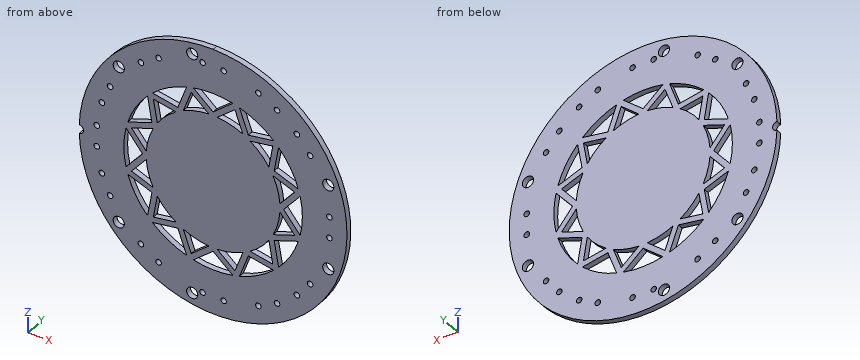
```python
from build123d import *

# Parameters (mm, degrees)
SKETCH2_R                = 88.9
BOSS_EXTRUDE1_DEPTH      = 3.175
SKETCH3_R                = 3.175
CUT_EXTRUDE1_DEPTH       = 3.175
SKETCH6_R                = 88.9
SKETCH6_R_2              = 76.2
CUT_EXTRUDE2_DEPTH       = 126.763669734
SKETCH7_R                = 1.5875
CUT_EXTRUDE3_DEPTH       = 108.809835474
SKETCH8_R                = 2.5
CUT_EXTRUDE4_DEPTH       = 108.809835474
CIRPATTERN1_COUNT        = 2
CIRPATTERN1_ANGLE        = 23
CIRPATTERN2_COUNT        = 2
CIRPATTERN2_ANGLE        = 57
CIRPATTERN3_COUNT        = 2
CIRPATTERN3_ANGLE        = 90
CIRPATTERN4_COUNT        = 2
CIRPATTERN6_COUNT        = 2
CIRPATTERN6_ANGLE        = 141
CIRPATTERN7_COUNT        = 2
CIRPATTERN7_ANGLE        = 118
MIRROR3_COPY_1_SKETCH_R  = 1.5875
MIRROR3_COPY_1_DEPTH     = 108.809835474
MIRROR3_COPY_2_SKETCH_R  = 1.5875
MIRROR3_COPY_2_DEPTH     = 108.809835474
MIRROR3_COPY_3_SKETCH_R  = 1.5875
MIRROR3_COPY_3_DEPTH     = 108.809835474
MIRROR3_COPY_4_SKETCH_R  = 1.5875
MIRROR3_COPY_4_DEPTH     = 108.809835474
MIRROR3_COPY_5_SKETCH_R  = 1.5875
MIRROR3_COPY_5_DEPTH     = 108.809835474
MIRROR3_COPY_6_SKETCH_R  = 1.5875
MIRROR3_COPY_6_DEPTH     = 108.809835474
MIRROR3_COPY_7_SKETCH_R  = 1.5875
MIRROR3_COPY_7_DEPTH     = 108.809835474
MIRROR3_COPY_8_SKETCH_R  = 1.5875
MIRROR3_COPY_8_DEPTH     = 108.809835474
MIRROR3_COPY_9_SKETCH_R  = 1.5875
MIRROR3_COPY_9_DEPTH     = 108.809835474
MIRROR3_COPY_10_SKETCH_R = 1.5875
MIRROR3_COPY_10_DEPTH    = 108.809835474
SKETCH11_R               = 50.8
SKETCH11_R_2             = 38.1
CUT_EXTRUDE6_DEPTH       = 108.809835474
EXTRUDE_THIN2_DEPTH      = 3.175


with BuildPart() as part:
    # Sketch2 → Boss-Extrude1 (new body)
    with BuildSketch(Plane(origin=(0, 0, 0), x_dir=(1, 0, 0), z_dir=(0, 1, 0))):
        with Locations(Location((0, 0, 0), (0, 0, 270))):
            Circle(SKETCH2_R)
    extrude(amount=BOSS_EXTRUDE1_DEPTH)

    # Sketch3 → Cut-Extrude1 (cut)
    with BuildSketch(Plane(origin=(0, 3.175, 0), x_dir=(1, 0, 0), z_dir=(0, 1, 0))):
        with Locations(Location((65.549718535, -24.13, 0), (0, 0, 270))):
            Circle(SKETCH3_R)
        with Locations(Location((65.549718535, 24.13, 0), (0, 0, 270))):
            Circle(SKETCH3_R)
        with Locations(Location((-53.672052261, 44.702721462, 0), (0, 0, 270))):
            Circle(SKETCH3_R)
        with Locations(Location((-11.877666274, 68.832721462, 0), (0, 0, 270))):
            Circle(SKETCH3_R)
        with Locations(Location((-11.877666274, -68.832721462, 0), (0, 0, 270))):
            Circle(SKETCH3_R)
        with Locations(Location((-53.672052261, -44.702721462, 0), (0, 0, 270))):
            Circle(SKETCH3_R)
    extrude(amount=-CUT_EXTRUDE1_DEPTH, mode=Mode.SUBTRACT)

    # Sketch6 → Cut-Extrude2 (cut, through all)
    with BuildSketch(Plane(origin=(0, 3.175, 0), x_dir=(1, 0, 0), z_dir=(0, 1, 0))):
        Circle(SKETCH6_R)
        with Locations(Location((0, 0, 0), (0, 0, 270))):
            Circle(SKETCH6_R_2, mode=Mode.SUBTRACT)
    extrude(amount=-CUT_EXTRUDE2_DEPTH, mode=Mode.SUBTRACT)

    # Sketch7 → Cut-Extrude3 (cut, symmetric)
    with BuildSketch(Plane(origin=(0, 3.175, 0), x_dir=(1, 0, 0), z_dir=(0, 1, 0))):
        with Locations(Location((-66.2, 6, 0), (0, 0, 270))):
            Circle(SKETCH7_R)
        with Locations(Location((-66.2, -6, 0), (0, 0, 270))):
            Circle(SKETCH7_R)
    cut_extrude3 = extrude(amount=CUT_EXTRUDE3_DEPTH, both=True, mode=Mode.SUBTRACT)

    # Sketch8 → Cut-Extrude4 (cut, through all)
    with BuildSketch(Plane(origin=(0, 3.175, 0), x_dir=(1, 0, 0), z_dir=(0, 1, 0))):
        with Locations((-76.2, 0)):
            Circle(SKETCH8_R)
    extrude(amount=-CUT_EXTRUDE4_DEPTH, mode=Mode.SUBTRACT)

    # CirPattern1: Cut-Extrude3 ×2 about axis
    cirpattern1_axis = Axis((0, 0, 0), (0, 1, 0))
    for i in range(1, CIRPATTERN1_COUNT):
        add(cut_extrude3.rotate(cirpattern1_axis, i * CIRPATTERN1_ANGLE / (CIRPATTERN1_COUNT - 1)), mode=Mode.SUBTRACT)

    # CirPattern2: Cut-Extrude3 ×2 about axis
    cirpattern2_axis = Axis((0, 0, 0), (0, 1, 0))
    for i in range(1, CIRPATTERN2_COUNT):
        add(cut_extrude3.rotate(cirpattern2_axis, i * CIRPATTERN2_ANGLE / (CIRPATTERN2_COUNT - 1)), mode=Mode.SUBTRACT)

    # CirPattern3: Cut-Extrude3 ×2 about axis
    cirpattern3_axis = Axis((0, 0, 0), (0, 1, 0))
    for i in range(1, CIRPATTERN3_COUNT):
        add(cut_extrude3.rotate(cirpattern3_axis, i * CIRPATTERN3_ANGLE / (CIRPATTERN3_COUNT - 1)), mode=Mode.SUBTRACT)

    # CirPattern4: Cut-Extrude3 ×2 about axis
    cirpattern4_axis = Axis((0, 0, 0), (0, 1, 0))
    for i in range(1, CIRPATTERN4_COUNT):
        add(cut_extrude3.rotate(cirpattern4_axis, i * 360 / CIRPATTERN4_COUNT), mode=Mode.SUBTRACT)

    # CirPattern6: Cut-Extrude3 ×2 about axis
    cirpattern6_axis = Axis((0, 0, 0), (0, 1, 0))
    for i in range(1, CIRPATTERN6_COUNT):
        add(cut_extrude3.rotate(cirpattern6_axis, i * CIRPATTERN6_ANGLE / (CIRPATTERN6_COUNT - 1)), mode=Mode.SUBTRACT)

    # CirPattern7: Cut-Extrude3 ×2 about axis
    cirpattern7_axis = Axis((0, 0, 0), (0, 1, 0))
    for i in range(1, CIRPATTERN7_COUNT):
        add(cut_extrude3.rotate(cirpattern7_axis, i * CIRPATTERN7_ANGLE / (CIRPATTERN7_COUNT - 1)), mode=Mode.SUBTRACT)

    # Mirror3 copy 1 sketch → Mirror3 copy 1 (cut, symmetric)
    with BuildSketch(Plane(origin=(0, 3.175, 0), x_dir=(0.9205048534524399, 0, 0.3907311284892746), z_dir=(0, 1, 0))):
        with Locations((-66.2, -6)):
            Circle(MIRROR3_COPY_1_SKETCH_R)
        with Locations((-66.2, 6)):
            Circle(MIRROR3_COPY_1_SKETCH_R)
    extrude(amount=MIRROR3_COPY_1_DEPTH, both=True, mode=Mode.SUBTRACT)

    # Mirror3 copy 2 sketch → Mirror3 copy 2 (cut, symmetric)
    with BuildSketch(Plane(origin=(0, 3.175, 0), x_dir=(1, 0, 0), z_dir=(0, 1, 0))):
        with Locations((-66.2, -6)):
            Circle(MIRROR3_COPY_2_SKETCH_R)
        with Locations((-66.2, 6)):
            Circle(MIRROR3_COPY_2_SKETCH_R)
    extrude(amount=MIRROR3_COPY_2_DEPTH, both=True, mode=Mode.SUBTRACT)

    # Mirror3 copy 3 sketch → Mirror3 copy 3 (cut, symmetric)
    with BuildSketch(Plane(origin=(0, 3.175, 0), x_dir=(0.5446390350150256, 0, 0.8386705679454249), z_dir=(0, 1, 0))):
        with Locations((-66.2, -6)):
            Circle(MIRROR3_COPY_3_SKETCH_R)
        with Locations((-66.2, 6)):
            Circle(MIRROR3_COPY_3_SKETCH_R)
    extrude(amount=MIRROR3_COPY_3_DEPTH, both=True, mode=Mode.SUBTRACT)

    # Mirror3 copy 4 sketch → Mirror3 copy 4 (cut, symmetric)
    with BuildSketch(Plane(origin=(0, 3.175, 0), x_dir=(1, 0, 0), z_dir=(0, 1, 0))):
        with Locations((-66.2, -6)):
            Circle(MIRROR3_COPY_4_SKETCH_R)
        with Locations((-66.2, 6)):
            Circle(MIRROR3_COPY_4_SKETCH_R)
    extrude(amount=MIRROR3_COPY_4_DEPTH, both=True, mode=Mode.SUBTRACT)

    # Mirror3 copy 5 sketch → Mirror3 copy 5 (cut, symmetric)
    with BuildSketch(Plane.ZX.offset(3.175)):
        with Locations((-66.2, -6)):
            Circle(MIRROR3_COPY_5_SKETCH_R)
        with Locations((-66.2, 6)):
            Circle(MIRROR3_COPY_5_SKETCH_R)
    extrude(amount=MIRROR3_COPY_5_DEPTH, both=True, mode=Mode.SUBTRACT)

    # Mirror3 copy 6 sketch → Mirror3 copy 6 (cut, symmetric)
    with BuildSketch(Plane(origin=(0, 3.175, 0), x_dir=(1, 0, 0), z_dir=(0, 1, 0))):
        with Locations((-66.2, -6)):
            Circle(MIRROR3_COPY_6_SKETCH_R)
        with Locations((-66.2, 6)):
            Circle(MIRROR3_COPY_6_SKETCH_R)
    extrude(amount=MIRROR3_COPY_6_DEPTH, both=True, mode=Mode.SUBTRACT)

    # Mirror3 copy 7 sketch → Mirror3 copy 7 (cut, symmetric)
    with BuildSketch(Plane(origin=(0, 3.175, 0), x_dir=(-0.7771459614569742, 0, 0.6293203910498333), z_dir=(0, 1, 0))):
        with Locations((-66.2, -6)):
            Circle(MIRROR3_COPY_7_SKETCH_R)
        with Locations((-66.2, 6)):
            Circle(MIRROR3_COPY_7_SKETCH_R)
    extrude(amount=MIRROR3_COPY_7_DEPTH, both=True, mode=Mode.SUBTRACT)

    # Mirror3 copy 8 sketch → Mirror3 copy 8 (cut, symmetric)
    with BuildSketch(Plane(origin=(0, 3.175, 0), x_dir=(1, 0, 0), z_dir=(0, 1, 0))):
        with Locations((-66.2, -6)):
            Circle(MIRROR3_COPY_8_SKETCH_R)
        with Locations((-66.2, 6)):
            Circle(MIRROR3_COPY_8_SKETCH_R)
    extrude(amount=MIRROR3_COPY_8_DEPTH, both=True, mode=Mode.SUBTRACT)

    # Mirror3 copy 9 sketch → Mirror3 copy 9 (cut, symmetric)
    with BuildSketch(Plane(origin=(0, 3.175, 0), x_dir=(-0.46947156278589486, 0, 0.8829475928589248), z_dir=(0, 1, 0))):
        with Locations((-66.2, -6)):
            Circle(MIRROR3_COPY_9_SKETCH_R)
        with Locations((-66.2, 6)):
            Circle(MIRROR3_COPY_9_SKETCH_R)
    extrude(amount=MIRROR3_COPY_9_DEPTH, both=True, mode=Mode.SUBTRACT)

    # Mirror3 copy 10 sketch → Mirror3 copy 10 (cut, symmetric)
    with BuildSketch(Plane(origin=(0, 3.175, 0), x_dir=(1, 0, 0), z_dir=(0, 1, 0))):
        with Locations((-66.2, -6)):
            Circle(MIRROR3_COPY_10_SKETCH_R)
        with Locations((-66.2, 6)):
            Circle(MIRROR3_COPY_10_SKETCH_R)
    extrude(amount=MIRROR3_COPY_10_DEPTH, both=True, mode=Mode.SUBTRACT)

    # Sketch11 → Cut-Extrude6 (cut, through all)
    with BuildSketch(Plane(origin=(0, 3.175, 0), x_dir=(1, 0, 0), z_dir=(0, 1, 0))):
        with Locations(Location((0, 0, 0), (0, 0, 270))):
            Circle(SKETCH11_R)
        with Locations(Location((0, 0, 0), (0, 0, 270))):
            Circle(SKETCH11_R_2, mode=Mode.SUBTRACT)
    extrude(amount=-CUT_EXTRUDE6_DEPTH, mode=Mode.SUBTRACT)


with BuildPart() as cut_extrude6_piece_1:
    # of the separate pieces the step leaves, piece 1, a body of its own (cut_extrude6_pieces)
    add(part.part.solids().sort_by_distance((-76.158989501, 0, 2.499663605))[0])



with BuildPart() as cut_extrude6_piece_2:
    # of the separate pieces the step leaves, piece 2, a body of its own (cut_extrude6_pieces)
    add(part.part.solids().sort_by_distance((0, 0, 38.1))[0])


with BuildPart() as cut_extrude6_piece_1_1:
    add(cut_extrude6_piece_1.part)

    add(cut_extrude6_piece_2.part)  # Extrude-Thin2 merges Cut-Extrude6 piece 2
    # Sketch12 → Extrude-Thin2 (add)
    with BuildSketch(Plane(origin=(0, 3.175, 0), x_dir=(1, 0, 0), z_dir=(0, 1, 0))):
        Polygon((-51.731661279, -13.861456863), (-34.786003978, -20.083708761), (-37.870204416, -37.870204416), (-20.083708761, -34.786003978), (-13.861456863, -51.731661279), (0, -40.167417522), (13.861456863, -51.731661279), (20.083708761, -34.786003978), (37.870204416, -37.870204416), (34.786003978, -20.083708761), (51.731661279, -13.861456863), (40.167417522, 0), (51.731661279, 13.861456863), (34.786003978, 20.083708761), (37.870204416, 37.870204416), (20.083708761, 34.786003978), (13.861456863, 51.731661279), (0, 40.167417522), (-13.861456863, 51.731661279), (-20.083708761, 34.786003978), (-37.870204416, 37.870204416), (-34.786003978, 20.083708761), (-51.731661279, 13.861456863), (-40.167417522, 0), align=None)
        Polygon((-46.406402672, -12.434558119), (-31.20513179, -18.016291239), (-33.971844552, -33.971844552), (-18.016291239, -31.20513179), (-12.434558119, -46.406402672), (0, -36.032582478), (12.434558119, -46.406402672), (18.016291239, -31.20513179), (33.971844552, -33.971844552), (31.20513179, -18.016291239), (46.406402672, -12.434558119), (36.032582478, 0), (46.406402672, 12.434558119), (31.20513179, 18.016291239), (33.971844552, 33.971844552), (18.016291239, 31.20513179), (12.434558119, 46.406402672), (0, 36.032582478), (-12.434558119, 46.406402672), (-18.016291239, 31.20513179), (-33.971844552, 33.971844552), (-31.20513179, 18.016291239), (-46.406402672, 12.434558119), (-36.032582478, 0), align=None, mode=Mode.SUBTRACT)
    extrude(amount=-EXTRUDE_THIN2_DEPTH)


solid = cut_extrude6_piece_1_1.part
```
Part model, mm, in its own coordinate system. Give positions to 0.01 mm unless a question says otherwise; leave off trailing zeros. Put each result on its own line as item: value. Start each with the question number.
Item 1: Wall check: L1, parallel to X at y = 2.3, z = -40; L2, parallel to X at y = 1.6, z = -67; L3, parallel to X at y = 0.4, z = -24.5. Give the ranges that are in metal, low to high. Write a range as [from, to].
Item 2: Cut at A-A (y = 0.9). State how many separate pieces and enclosed holes the cut face has, then the cut area to 3 significant figures.
Item 3: Pin check, flat tip, straight feed: pin 1 Ø5.5 at (x, z) = (-53.67, 44.7) entering from +Y. Stop position of the tip, or through.
Answer list:
1. L1: x = [-64.86, -31.32], [-18.17, -14.79], [-4.76, 4.76], [14.79, 18.17], [31.32, 64.86]
1. L2: x = [-36.3, -14.47], [-9.29, -7.37], [-4.63, 4.63], [7.37, 36.3]
1. L3: x = [-72.15, -44.5], [-35.55, -32.33], [-29.18, 29.18], [32.33, 35.55], [44.5, 62.4], [68.7, 72.15]
2. separate pieces: 1
2. enclosed holes: 54
2. area: 15,500 mm2
3. pin 1: passes through
